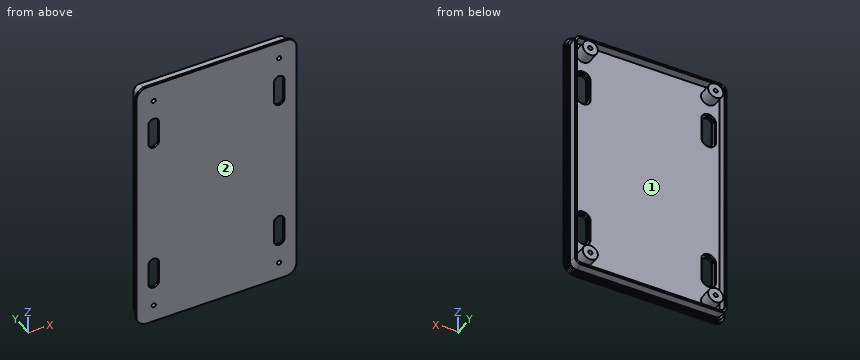
from build123d import *

# Parameters (mm, degrees)
SKETCH1_W           = 76
SKETCH1_H           = 123
SKETCH1_R           = 3.6
BOSS_EXTRUDE2_DEPTH = 2
SKETCH1_4_R         = 3.6
BOSS_EXTRUDE3_DEPTH = 6
FILLET1_R           = 5
CUT_EXTRUDE1_DEPTH  = 73.541367508
SKETCH3_R           = 1
CUT_EXTRUDE2_DEPTH  = 73.734104793
CUT_EXTRUDE4_DEPTH  = 1
BOSS_EXTRUDE4_DEPTH = 4


with BuildPart() as part:
    # Sketch1 → Boss-Extrude2 (new body)
    with BuildSketch(Plane(origin=(0, 0, 0), x_dir=(1, 0, 0), z_dir=(0, 1, 0))):
        Rectangle(SKETCH1_W, SKETCH1_H)
        with Locations((-29.8, -53.3)):
            Circle(SKETCH1_R, mode=Mode.SUBTRACT)
        with Locations((29.8, -53.3)):
            Circle(SKETCH1_R, mode=Mode.SUBTRACT)
        with Locations((29.8, 53.3)):
            Circle(SKETCH1_R, mode=Mode.SUBTRACT)
        with Locations((-29.8, 53.3)):
            Circle(SKETCH1_R, mode=Mode.SUBTRACT)
        with Locations((-29.8, -53.3)):
            Circle(SKETCH1_R)
        with Locations((29.8, -53.3)):
            Circle(SKETCH1_R)
        with Locations((-29.8, 53.3)):
            Circle(SKETCH1_R)
        with Locations((29.8, 53.3)):
            Circle(SKETCH1_R)
    extrude(amount=-BOSS_EXTRUDE2_DEPTH)

    # Sketch1_4 → Boss-Extrude3 (add)
    with BuildSketch(Plane(origin=(0, 0, 0), x_dir=(1, 0, 0), z_dir=(0, 1, 0))):
        with Locations(Location((-29.8, -53.3, 0), (0, 0, 270))):
            Circle(SKETCH1_4_R)
        with Locations(Location((29.8, -53.3, 0), (0, 0, 270))):
            Circle(SKETCH1_4_R)
        with Locations(Location((-29.8, 53.3, 0), (0, 0, 270))):
            Circle(SKETCH1_4_R)
        with Locations(Location((29.8, 53.3, 0), (0, 0, 270))):
            Circle(SKETCH1_4_R)
    extrude(amount=BOSS_EXTRUDE3_DEPTH)

    # Fillet1
    fillet1_edges = [part.edges().sort_by_distance(p)[0] for p in [
        (-38, -1, 61.5),
        (-38, -1, -61.5),
        (38, -1, -61.5),
        (38, -1, 61.5),
    ]]
    fillet(fillet1_edges, radius=FILLET1_R)

    # Sketch2 → Cut-Extrude1 (cut, through all)
    with BuildSketch(Plane(origin=(0, 0, 0), x_dir=(1, 0, 0), z_dir=(0, 1, 0))):
        with BuildLine():
            Line((-27.3, 41.5), (-27.3, 31.5))
            ThreePointArc((-27.3, 31.5), (-29.8, 29), (-32.3, 31.5))
            Line((-32.3, 31.5), (-32.3, 41.5))
            ThreePointArc((-32.3, 41.5), (-29.8, 44), (-27.3, 41.5))
        make_face()
        with BuildLine():
            Line((27.3, 41.5), (27.3, 31.5))
            ThreePointArc((27.3, 31.5), (29.8, 29), (32.3, 31.5))
            Line((32.3, 31.5), (32.3, 41.5))
            ThreePointArc((32.3, 41.5), (29.8, 44), (27.3, 41.5))
        make_face()
        with BuildLine():
            Line((-27.3, -41.5), (-27.3, -31.5))
            ThreePointArc((-27.3, -31.5), (-29.8, -29), (-32.3, -31.5))
            Line((-32.3, -31.5), (-32.3, -41.5))
            ThreePointArc((-32.3, -41.5), (-29.8, -44), (-27.3, -41.5))
        make_face()
        with BuildLine():
            Line((27.3, -41.5), (27.3, -31.5))
            ThreePointArc((27.3, -31.5), (29.8, -29), (32.3, -31.5))
            Line((32.3, -31.5), (32.3, -41.5))
            ThreePointArc((32.3, -41.5), (29.8, -44), (27.3, -41.5))
        make_face()
    extrude(amount=-CUT_EXTRUDE1_DEPTH, mode=Mode.SUBTRACT)

    # Sketch3 → Cut-Extrude2 (cut, through all)
    with BuildSketch(Plane(origin=(0, 6, 0), x_dir=(1, 0, 0), z_dir=(0, 1, 0))):
        with Locations(Location((-29.8, -53.3, 0), (0, 0, 270))):
            Circle(SKETCH3_R)
        with Locations(Location((29.8, -53.3, 0), (0, 0, 90))):
            Circle(SKETCH3_R)
        with Locations(Location((29.8, 53.3, 0), (0, 0, 270))):
            Circle(SKETCH3_R)
        with Locations(Location((-29.8, 53.3, 0), (0, 0, 90))):
            Circle(SKETCH3_R)
    extrude(amount=-CUT_EXTRUDE2_DEPTH, mode=Mode.SUBTRACT)

    # Sketch4 → Cut-Extrude4 (cut)
    with BuildSketch(Plane(origin=(0, 0, 0), x_dir=(1, 0, 0), z_dir=(0, 1, 0))):
        with BuildLine():
            ThreePointArc((38, 56.5), (36.535533906, 60.035533906), (33, 61.5))
            Line((33, 61.5), (-33, 61.5))
            ThreePointArc((-33, 61.5), (-36.535533906, 60.035533906), (-38, 56.5))
            Line((-38, 56.5), (-38, -56.5))
            ThreePointArc((-38, -56.5), (-36.535533906, -60.035533906), (-33, -61.5))
            Line((-33, -61.5), (33, -61.5))
            ThreePointArc((33, -61.5), (36.535533906, -60.035533906), (38, -56.5))
            Line((38, -56.5), (38, 56.5))
        make_face()
        with BuildLine():
            ThreePointArc((-37, -56.5), (-35.828427125, -59.328427125), (-33, -60.5))
            Line((-33, -60.5), (33, -60.5))
            ThreePointArc((33, -60.5), (35.828427125, -59.328427125), (37, -56.5))
            Line((37, -56.5), (37, 56.5))
            ThreePointArc((37, 56.5), (35.828427125, 59.328427125), (33, 60.5))
            Line((33, 60.5), (-33, 60.5))
            ThreePointArc((-33, 60.5), (-35.828427125, 59.328427125), (-37, 56.5))
            Line((-37, 56.5), (-37, -56.5))
        make_face(mode=Mode.SUBTRACT)
        with BuildLine():
            Line((-33.3, -31.5), (-33.3, -41.5))
            ThreePointArc((-33.3, -41.5), (-29.8, -45), (-26.3, -41.5))
            Line((-26.3, -41.5), (-26.3, -31.5))
            ThreePointArc((-26.3, -31.5), (-29.8, -28), (-33.3, -31.5))
        make_face()
        with BuildLine():
            Line((-27.3, -31.5), (-27.3, -41.5))
            ThreePointArc((-27.3, -41.5), (-29.8, -44), (-32.3, -41.5))
            Line((-32.3, -41.5), (-32.3, -31.5))
            ThreePointArc((-32.3, -31.5), (-29.8, -29), (-27.3, -31.5))
        make_face(mode=Mode.SUBTRACT)
        with BuildLine():
            Line((33.3, -41.5), (33.3, -31.5))
            ThreePointArc((33.3, -31.5), (29.8, -28), (26.3, -31.5))
            Line((26.3, -31.5), (26.3, -41.5))
            ThreePointArc((26.3, -41.5), (29.8, -45), (33.3, -41.5))
        make_face()
        with BuildLine():
            Line((32.3, -31.5), (32.3, -41.5))
            ThreePointArc((32.3, -41.5), (29.8, -44), (27.3, -41.5))
            Line((27.3, -41.5), (27.3, -31.5))
            ThreePointArc((27.3, -31.5), (29.8, -29), (32.3, -31.5))
        make_face(mode=Mode.SUBTRACT)
        with BuildLine():
            Line((33.3, 31.5), (33.3, 41.5))
            ThreePointArc((33.3, 41.5), (29.8, 45), (26.3, 41.5))
            Line((26.3, 41.5), (26.3, 31.5))
            ThreePointArc((26.3, 31.5), (29.8, 28), (33.3, 31.5))
        make_face()
        with BuildLine():
            Line((27.3, 31.5), (27.3, 41.5))
            ThreePointArc((27.3, 41.5), (29.8, 44), (32.3, 41.5))
            Line((32.3, 41.5), (32.3, 31.5))
            ThreePointArc((32.3, 31.5), (29.8, 29), (27.3, 31.5))
        make_face(mode=Mode.SUBTRACT)
        with BuildLine():
            Line((-33.3, 41.5), (-33.3, 31.5))
            ThreePointArc((-33.3, 31.5), (-29.8, 28), (-26.3, 31.5))
            Line((-26.3, 31.5), (-26.3, 41.5))
            ThreePointArc((-26.3, 41.5), (-29.8, 45), (-33.3, 41.5))
        make_face()
        with BuildLine():
            Line((-32.3, 31.5), (-32.3, 41.5))
            ThreePointArc((-32.3, 41.5), (-29.8, 44), (-27.3, 41.5))
            Line((-27.3, 41.5), (-27.3, 31.5))
            ThreePointArc((-27.3, 31.5), (-29.8, 29), (-32.3, 31.5))
        make_face(mode=Mode.SUBTRACT)
    extrude(amount=-CUT_EXTRUDE4_DEPTH, mode=Mode.SUBTRACT)

    # Sketch5 → Boss-Extrude4 (add)
    with BuildSketch(Plane(origin=(0, 0, 0), x_dir=(1, 0, 0), z_dir=(0, 1, 0))):
        with BuildLine():
            Line((-36, 56.5), (-36, -56.5))
            ThreePointArc((-36, -56.5), (-35.121320344, -58.621320344), (-33, -59.5))
            Line((-33, -59.5), (33, -59.5))
            ThreePointArc((33, -59.5), (35.121320344, -58.621320344), (36, -56.5))
            Line((36, -56.5), (36, 56.5))
            ThreePointArc((36, 56.5), (35.121320344, 58.621320344), (33, 59.5))
            Line((33, 59.5), (-33, 59.5))
            ThreePointArc((-33, 59.5), (-35.121320344, 58.621320344), (-36, 56.5))
        make_face()
        with BuildLine():
            Line((-35, 56.5), (-35, -56.5))
            ThreePointArc((-35, -56.5), (-34.414213562, -57.914213562), (-33, -58.5))
            Line((-33, -58.5), (33, -58.5))
            ThreePointArc((33, -58.5), (34.414213562, -57.914213562), (35, -56.5))
            Line((35, -56.5), (35, 56.5))
            ThreePointArc((35, 56.5), (34.414213562, 57.914213562), (33, 58.5))
            Line((33, 58.5), (-33, 58.5))
            ThreePointArc((-33, 58.5), (-34.414213562, 57.914213562), (-35, 56.5))
        make_face(mode=Mode.SUBTRACT)
    extrude(amount=BOSS_EXTRUDE4_DEPTH)


solid = part.part
Geometry check sheet. Reference: the model listing, model coordinates, mm. Face numbers are marked on the shaded views. Coordinates: 2 decimals unless noted, no trailing zeros. Order: outer loops, then holes, each group sorted by start corner. A loop starts at its lowest first (then second) coordinate and runs counter-clockwise, first axis right, second up. Notation, with made-up numbers: (65.25, -20) -> (85.25, -20) arc R11 cw to (85.25, 1) -> close; hole circle Ø7 at (66.5, 88.5). An arc over 180 degrees is marked (long way). Use a Markdown table: item, result. Add a question column.
1. Mould release check, pull along Z, two halves, no side actions. Record for the marked faces 1 and 2: pulls with the +Z half, pulls with the -Z half, needs draft (parallel to the pull), parting line crosses it, or undercut.
2. Cross-section at D-D (z = 20.5). Enter the section's corners in (x, y), and give its area (3 significant figures).
3. Material ranges on L1, parallel to X at y = 1, z = 53.3; L2, parallel to X at y = 3.75, z = 35.5; L3, parallel to Z at x = -33, y = 1.5, recorded low to high.
4. Cross-section at A-A (y = 2.5). Give the number of separate pieces and of enclosed holes in the cut face, and give its area (3 significant figures).
5. Go/stop test with flat-tipped pins: pin 1 Ø3 at (y, z) = (-0.5, 46) entering from -X; pin 2 Ø1 at (y, z) = (2.5, 49) entering from -X; pin 3 Ø3 at (x, y) = (-12, 3) entering from -Z; pin 4 Ø0.8 at (y, z) = (-0.5, -34.5) entering from +X. Record where each tip stops, or that it passes through.
6. Cross-section at C-C (x = -22). Enter the section's corners in (y, z).
Filled sheet:
| question | item | result |
|---|---|---|
| 1 | face 1 | undercut |
| 1 | face 2 | needs draft |
| 2 | outline | (-38, -2) -> (38, -2) -> (38, -1) -> (37, -1) -> (37, 0) -> (36, 0) -> (36, 4) -> (35, 4) -> (35, 0) -> (-35, 0) -> (-35, 4) -> (-36, 4) -> (-36, 0) -> (-37, 0) -> (-37, -1) -> (-38, -1) -> close |
| 2 | area | 158 mm2 |
| 3 | L1 | -36 to -35, -33.4 to -30.8, -28.8 to -26.2, 26.2 to 28.8, 30.8 to 33.4, 35 to 36 |
| 3 | L2 | -36 to -35, 35 to 36 |
| 3 | L3 | -59.5 to -58.5, -54.95 to -51.65, 51.65 to 54.95, 58.5 to 59.5 |
| 4 | separate pieces | 5 |
| 4 | enclosed holes | 5 |
| 4 | area | 524 mm2 |
| 5 | pin 1 | x = -38 |
| 5 | pin 2 | x = -36 |
| 5 | pin 3 | z = -59.5 |
| 5 | pin 4 | x = 37 |
| 6 | outline | (-2, -61.5) -> (-1, -61.5) -> (-1, -60.5) -> (0, -60.5) -> (0, -59.5) -> (4, -59.5) -> (4, -58.5) -> (0, -58.5) -> (0, 58.5) -> (4, 58.5) -> (4, 59.5) -> (0, 59.5) -> (0, 60.5) -> (-1, 60.5) -> (-1, 61.5) -> (-2, 61.5) -> close |
